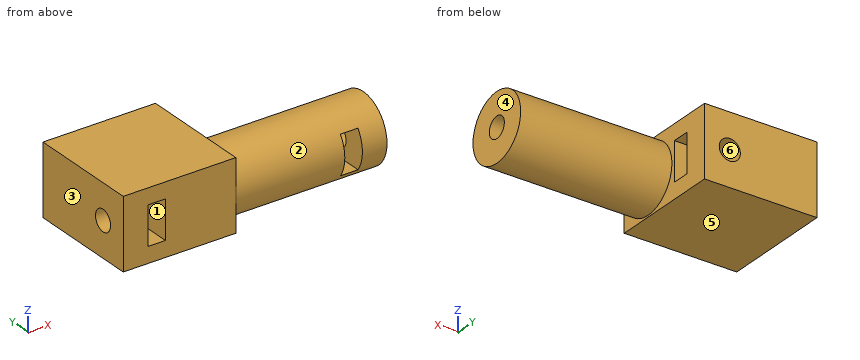
from build123d import *

# Parameters (mm, degrees)
SKETCH1_W           = 16
SKETCH1_H           = 16
BOSS_EXTRUDE1_DEPTH = 10
SKETCH2_R           = 1.5
CUT_EXTRUDE1_DEPTH  = 6
SKETCH3_R           = 1.5
CUT_EXTRUDE2_DEPTH  = 6
CUT_EXTRUDE3_START  = -3.5
CUT_EXTRUDE3_DEPTH  = 2.5
CUT_EXTRUDE5_START  = -3.5
SKETCH6_W           = 5.5
SKETCH6_H           = 8.06
CUT_EXTRUDE5_DEPTH  = 2.5
CUT_EXTRUDE6_START  = -3.5
SKETCH7_W           = 7.078957324
SKETCH7_H           = 5.4986679
CUT_EXTRUDE6_DEPTH  = 2.5
SKETCH9_R           = 4.75
BOSS_EXTRUDE2_DEPTH = 21.5
SKETCH10_R          = 1.5
CUT_EXTRUDE7_DEPTH  = 6
CUT_EXTRUDE9_START  = -3.5
SKETCH11_R          = 1.5
CUT_EXTRUDE9_DEPTH  = 2.5


with BuildPart() as part:
    # Sketch1 → Boss-Extrude1 (new body)
    with BuildSketch(Plane.XY):
        Rectangle(SKETCH1_W, SKETCH1_H)
    extrude(amount=BOSS_EXTRUDE1_DEPTH)

    # Sketch2 → Cut-Extrude1 (cut)
    with BuildSketch(Plane.ZY.offset(8)):
        with Locations(Location((5, -3.97, 0), (0, 0, 270))):
            Circle(SKETCH2_R)
    extrude(amount=-CUT_EXTRUDE1_DEPTH, mode=Mode.SUBTRACT)

    # Sketch3 → Cut-Extrude2 (cut)
    with BuildSketch(Plane(origin=(0, 8, 0), x_dir=(1, 0, 0), z_dir=(0, 1, 0))):
        with Locations(Location((4.4, -5, 0), (0, 0, 270))):
            Circle(SKETCH3_R)
    extrude(amount=-CUT_EXTRUDE2_DEPTH, mode=Mode.SUBTRACT)

    # Sketch4 → Cut-Extrude3 (cut)
    with BuildSketch(Plane.ZY.offset(8).offset(CUT_EXTRUDE3_START)):
        Polygon((7.75, -2.38228676), (5, -0.794573519), (2.25, -2.38228676), (2.25, -5.55771324), (5, -7.145426481), (7.75, -5.55771324), align=None)
    extrude(amount=-CUT_EXTRUDE3_DEPTH, mode=Mode.SUBTRACT)

    # Sketch6 → Cut-Extrude5 (cut)
    with BuildSketch(Plane.ZY.offset(8).offset(CUT_EXTRUDE5_START)):
        with Locations((5, -8)):
            Rectangle(SKETCH6_W, SKETCH6_H)
    extrude(amount=-CUT_EXTRUDE5_DEPTH, mode=Mode.SUBTRACT)

    # Sketch7 → Cut-Extrude6 (cut)
    with BuildSketch(Plane(origin=(0, 8, 0), x_dir=(1, 0, 0), z_dir=(0, 1, 0)).offset(CUT_EXTRUDE6_START)):
        Polygon((7.574657392, -5.069884021), (6.047850034, -2.285608061), (2.873192642, -2.21572404), (1.225342608, -4.930115979), (2.752149966, -7.714391939), (5.926807358, -7.78427596), align=None)
        with Locations((8, -5)):
            Rectangle(SKETCH7_W, SKETCH7_H)
    extrude(amount=-CUT_EXTRUDE6_DEPTH, mode=Mode.SUBTRACT)

    # Sketch9 → Boss-Extrude2 (add)
    with BuildSketch(Plane(origin=(8, 0, 0), x_dir=(0, 0, -1), z_dir=(1, 0, 0))):
        with Locations(Location((-4.985464698, -3.25, 0), (0, 0, 270))):
            Circle(SKETCH9_R)
    extrude(amount=BOSS_EXTRUDE2_DEPTH)

    # Sketch10 → Cut-Extrude7 (cut)
    with BuildSketch(Plane(origin=(29.5, 0, 0), x_dir=(0, 0, -1), z_dir=(1, 0, 0))):
        with Locations(Location((-4.985464698, -3.25, 0), (0, 0, 90))):
            Circle(SKETCH10_R)
    extrude(amount=-CUT_EXTRUDE7_DEPTH, mode=Mode.SUBTRACT)

    # Sketch11 → Cut-Extrude9 (cut)
    with BuildSketch(Plane(origin=(29.5, 0, 0), x_dir=(0, 0, -1), z_dir=(1, 0, 0)).offset(CUT_EXTRUDE9_START)):
        with BuildLine():
            Line((-2.31047639, -1.538926979), (-5.129803248, -0.07785566))
            Line((-5.129803248, -0.07785566), (-7.804791556, -1.78892868))
            Line((-7.804791556, -1.78892868), (-7.738307115, -3.250064634))
            Line((-7.738307115, -3.250064634), (-7.738307115, -7.120963527))
            ThreePointArc((-7.738307115, -7.120963527), (-4.988950766, -7.999998721), (-2.238307115, -7.125000027))
            Line((-2.238307115, -7.125000027), (-2.238307115, -3.12499915))
            Line((-2.238307115, -3.12499915), (-2.31047639, -1.538926979))
        make_face()
        with Locations(Location((-4.985464698, -3.25, 0), (0, 0, 90))):
            Circle(SKETCH11_R, mode=Mode.SUBTRACT)
    extrude(amount=-CUT_EXTRUDE9_DEPTH, mode=Mode.SUBTRACT)


solid = part.part
Input: part model. Units: mm. Frame: model coordinates. Face numbers are marked on the shaded views. A direction names the side the tool comes from. Give positions to 0.01 mm unless a question says otherwise; leave off trailing zeros. Write each loop counter-clockwise with the first axis right and the second up, starting at its lowest first coordinate (ties: lowest second). Pieces come first, ordered by that corner, then holes.
Q1. Set-up query: the marked faces 1, 2 and 3. Return all of +Z, -Z, +X, -X, +Y, -Y with unobstructed straight access to the full face (end or side cutting, diameter ignored); none if empty.
Q2. Section D-D, the plane y = 0.75. Output: boundary loops of the cut face in (x, z), plus the area to 3 significant figures.
Q3. Section A-A, the plane x = -2.5. Output: boundary loops of the cut face in (y, z), plus the area to 3 significant figures.
Q4. Section B-B, the plane x = 2. Output: boundary loops of the cut face in (y, z), plus the area to 3 significant figures.
Q5. First-contact query: P1, Ø3, axis at x = 24, y = -4, coming from the +Z side; P2, Ø1.8, axis at x = 4.4, z = 5, coming from the +Y side; P3, Ø2.5, axis at y = -3.25, z = 4.99, coming from the +X side. Flat tips, straight axial feed; report the tip coordinate or a pass-through.
Q6. Material intervals for probe 1 along X at (y, z) = (-6.5, 4); probe 2 along Y at (x, z) = (-7.05, 5); probe 3 along Z at (x, y) = (-6.5, -3.97), sorted ascending.
Q7. Pull-direction query (X, two-part tool) for the marked faces 4, 5 and 6; classes: pulls with the +X half, pulls with the -X half, needs draft (parallel to the pull), parting line crosses it, or undercut.
Q8. Section C-C, the plane z = 1.25. Output: boundary loops of the cut face in (x, y), plus the area to 3 significant figures.
Filled in:
1. face 1: -Y
1. face 2: +X
1. face 3: +Z, -Z, -X, +Y, -Y
2. outline: (-8, 0) - (8, 0) - (8, 2.42) - (29.5, 2.42) - (29.5, 7.55) - (8, 7.55) - (8, 10) - (-8, 10) - close
2. area: 270 mm2
3. outline: (-8, 0) - (8, 0) - (8, 10) - (-8, 10) - (-8, 7.75) - (-2.38, 7.75) - (-0.79, 5) - (-2.38, 2.25) - (-8, 2.25) - close
3. area: 125 mm2
4. outline: (-8, 0) - (8, 0) - (8, 10) - (-8, 10) - close; hole (2, 3.65) - (4.5, 3.65) - (4.5, 6.34) - (2, 6.34) - close
4. area: 153 mm2
5. P1: stops at z = 9.74
5. P2: stops at y = 2
5. P3: stops at x = 23.5
6. probe 1: x = -8 to -4.5, -2 to 23.5, 26 to 29.5
6. probe 2: y = -8 to -5.47, -2.47 to 8
6. probe 3: z = 0 to 3.5, 6.5 to 10
7. face 4: pulls with the +X half
7. face 5: needs draft
7. face 6: undercut
8. outline: (-8, -8) - (8, -8) - (8, -6.18) - (29.5, -6.18) - (29.5, -0.32) - (8, -0.32) - (8, 8) - (-8, 8) - close
8. area: 382 mm2
